Design review of the part built by this model. Coordinates are the model's own, in mm. A direction names the side the tool comes from. Give positions to 0.01 mm unless a question says otherwise; leave off trailing zeros. Order: outer loops, then holes, each group sorted by start corner. A loop starts at its lowest first (then second) coordinate and runs counter-clockwise, first axis right, second up.
Autodesk Inventor part; units mm, degrees
ref_plane "mdk_2_XY" through (0, 0, 0) normal (1, 0, 0) x (0, 0, -1)
ref_plane "mdk_2_YZ" through (0, 0, 0) normal (0, 0, -1) x (0, 1, 0)
ref_plane "mdk_2_ZX" through (0, 0, 0) normal (0, 1, 0) x (1, 0, 0)
sketch "Sketch_1" plane through (0, 0, 0) normal (1, 0, 0) x (0, 1, 0)
  line L0 (10.2835, 9.5) -> (-10.2835, 9.5)
  arc A0 (-10.2835, 9.5) -> (-10.2835, -9.5) centre (0, 0) ccw
  line L1 (-10.2835, -9.5) -> (10.2835, -9.5)
  arc A1 (10.2835, -9.5) -> (10.2835, 9.5) centre (0, 0) ccw
extrude "Extrusion1" add sketch "Sketch_1" along normal blind 5
sketch "Sketch_9" plane through (0, 0, 0) normal (0, 0, 1) x (1, 0, 0)
  line L0 (50, 0) -> (-50, 0)
  line L1 (0, 13.2) -> (1, 14.2)
  line L2 (1, 14.2) -> (0, 14.2)
  line L3 (0, 14.2) -> (0, 13.2)
revolve "Revolution1" cut sketch "Sketch_9" angle 360 about axis through (50, 0, 0) along (1, 0, 0)
sketch "Sketch_10" plane through (0, 0, 0) normal (0, 0, 1) x (1, 0, 0)
  line L0 (50, 0) -> (-50, 0)
  line L1 (4, 14.2) -> (5, 13.2)
  line L2 (5, 13.2) -> (5, 14.2)
  line L3 (5, 14.2) -> (4, 14.2)
revolve "Revolution2" cut sketch "Sketch_10" angle 360 about axis through (50, 0, 0) along (1, 0, 0)
sketch "Sketch4" plane through (5, 0, 0) normal (1, 0, 0) x (0, 0, -1)
  point P0 (-5.5, 9.5263)
hole "Hole1" at (5, 9.5263, 5.5) direction (-1, 0, 0) diameter 3.4 depth 5
sketch "Sketch5" plane through (5, 0, 0) normal (1, 0, 0) x (0, 0, -1)
  point P0 (5.5, -9.5263)
hole "Hole2" at (5, -9.5263, -5.5) direction (-1, 0, 0) diameter 3.4 depth 5
sketch "Sketch6" plane through (5, 0, 0) normal (1, 0, 0) x (0, 0, -1)
  point P0 (5.5, 9.5263)
hole "Hole3" at (5, 9.5263, -5.5) direction (-1, 0, 0) diameter 3.4 depth 5
sketch "Sketch7" plane through (5, 0, 0) normal (1, 0, 0) x (0, 0, -1)
  point P0 (-5.5, -9.5263)
hole "Hole4" at (5, -9.5263, 5.5) direction (-1, 0, 0) diameter 3.4 depth 5
sketch "Sketch8" plane through (0, 0, 0) normal (-1, 0, 0) x (0, 0, 1)
  point P0 (0, 0)
hole "Hole5" at (0, 0, 0) direction (1, 0, 0) diameter 8 depth 5
sketch "Sketch_14" plane through (0, 0, 0) normal (0, 0, 1) x (1, 0, 0)
  line L0 (50, 0) -> (-50, 0)
  line L1 (5, 7.2) -> (5, 4)
  line L2 (5, 4) -> (22, 4)
  line L3 (22, 4) -> (22, 6.5)
  line L4 (22, 6.5) -> (21, 7.5)
  line L5 (21, 7.5) -> (8, 7.5)
  line L6 (8, 7.5) -> (8, 7.2)
  line L7 (8, 7.2) -> (5, 7.2)
revolve "Revolution3" add sketch "Sketch_14" angle 360 about axis through (50, 0, 0) along (1, 0, 0)
sketch "Sketch_5" plane through (0, 0, 0) normal (1, 0, 0) x (0, 1, 0)
  circle A0 centre (0, 0) radius 6
extrude "Extrusion2" cut sketch "Sketch_5" along normal blind 4
sketch "Sketch_6" plane through (22, 0, 0) normal (1, 0, 0) x (0, 0, -1)
  circle A0 centre (0, 0) radius 6
extrude "Extrusion3" cut sketch "Sketch_6" against normal blind 4
ref_plane "mdk_2_XY" through (0, 0, 0) normal (1, 0, 0) x (0, 0, -1)
ref_plane "mdk_2_YZ" through (0, 0, 0) normal (0, 0, -1) x (0, 1, 0)
ref_plane "mdk_2_ZX" through (0, 0, 0) normal (0, 1, 0) x (1, 0, 0)
properties part number "MDK 0802-30420 Nut"
1. For pin 1 (4 mm diameter, centred on y = 9.53, z = 5.5, fed in from +X); pin 2 (9.5 mm diameter, centred on y = 0, z = 0, fed in from +X); pin 3 (4 mm diameter, centred on x = 14.5, y = 7.5, fed in from -Z), all flat-tipped, find the tip position at first contact; note any pin that passes through.
Recorded:
pin 1: stops at x = 5
pin 2: stops at x = 18
pin 3: stops at z = -5.1
2. For line 1 along Y through (x, z) = (1.75, -5.5); line 2 along Z through (x, y) = (15, 0); line 3 along Z through (x, y) = (0.8, 0), list the stretches that pass through material, from the lowest coordinate up.
Recorded:
line 1: y = -12.87 to -11.23, -7.83 to -2.4, 2.4 to 7.83, 11.23 to 12.87
line 2: z = -7.5 to -4, 4 to 7.5
line 3: z = -9.5 to -6, 6 to 9.5
3. Take a section at D-D (x = 12.25). State the section outline as (y, z) points, then the cut area to 3 significant figures.
Recorded:
outline: circle Ø15 at (0, 0); hole circle Ø8 at (0, 0)
area: 126 mm2
4. Take a section at B-B (x = 7). State the section outline as (y, z) points, then the cut area to 3 significant figures.
Recorded:
outline: circle Ø14.4 at (0, 0); hole circle Ø8 at (0, 0)
area: 113 mm2
5. Take a section at A-A (x = 1.75). State the section outline as (y, z) points, then the cut area to 3 significant figures.
Recorded:
outline: (-10.28, -9.5) - (10.28, -9.5) arc R14 ccw to (10.28, 9.5) - (-10.28, 9.5) arc R14 ccw to start; hole circle Ø3.4 at (-9.53, -5.5); hole circle Ø3.4 at (-9.53, 5.5); hole circle Ø12 at (0, 0); hole circle Ø3.4 at (9.53, -5.5); hole circle Ø3.4 at (9.53, 5.5)
area: 338 mm2
6. Draft analysis for pull direction X (two halves, no side actions). For faces 4 (the face through (0.14, -13.34, 0.15)), 5 (the face through (14.409, -7.493, -0.33)), 6 (the face through (4.86, -13.34, -0.15)), 7 (the face through (6.48, 6.87, -2.16)), state which applies: pulls with the +X half, pulls with the -X half, needs draft (parallel to the pull), parting line crosses it, or undercut.
Recorded:
face 4: pulls with the -X half
face 5: needs draft
face 6: pulls with the +X half
face 7: undercut
7. Take a section at C-C (z = -5.5). State how many separate pieces and enclosed holes the cut face has, then the cut area to 3 significant figures.
Recorded:
separate pieces: 3
enclosed holes: 0
area: 224 mm2
8. Machinability: for faces 1 (the face through (2.46, -11.21, 5.72)), 2 (the face through (2, -6, 0)), 3 (the face through (20, 0, 6)), which of the approach directions +Z, -Z, +X, -X, +Y, -Y give a long, thin tool a straight path to every point of the face, cutting with its end or side? Answer none if there is none.
Recorded:
face 1: +X, -X
face 2: -X
face 3: +X
